from build123d import *

# Parameters (mm, degrees)
F0_R     = 63.5
F1_DEPTH = 254
F2_R     = 31.75
F3_DEPTH = 50.8


# Not quite as in the source:
# - a pattern or mirror of a feature is missing from the dataset's text; its kind, count and spacing are read off the source's solid


with BuildPart() as f1:
    # F0 (on Front) → F1 (new body)
    with BuildSketch(Plane.XZ):
        Circle(F0_R)
    extrude(amount=F1_DEPTH)

    # F2 (on face) → F3 (join)
    with BuildSketch(Plane.XZ.offset(254)):
        Circle(F2_R)
    f3 = extrude(amount=F3_DEPTH)

    # F3_copies: F3 across plane
    add(f3.mirror(Plane.ZX.offset(-127)))


solid = f1.part
Verification items for the finished model (mm, model axes). A direction names the side the tool comes from. Coordinates: 2 decimals unless noted, no trailing zeros. Order: outer loops, then holes, each group sorted by start corner. A loop starts at its lowest first (then second) coordinate and runs counter-clockwise, first axis right, second up. Notation, with made-up numbers: M -17,22 L 3,22 A21 cw 3,52 Z; hole C -22,53 d8. An arc over 180 degrees is marked long. One line per item, written item: value. Start each with the question number.
Item 1: Sectioned sample at D-D on x = -47.5. Record the cut outline in (y, z), then the cut area to 3 significant figures.
Item 2: Thickness scan on probe 1 along Z at (x, y) = (-1, -238); probe 2 along Y at (x, z) = (27, 55.5); probe 3 along X at (y, z) = (-133, 1.5). Record the ranges inside material, lowest first.
Item 3: Sectioned sample at C-C on y = -102.5. Record the cut outline in (x, z), then the cut area to 3 significant figures.
Item 4: Access from +Z, -Z, +X, -X, +Y, -Y to the whole of each face (thin tool, end or side, straight path). Record for faces 1 (the flat face through (0, 50.8, 0)), 2 (the cylindrical face through (-6.883, -279.044, -30.995)), 3 (the flat face through (13.2, 0, 29.1)).
Item 5: Sectioned sample at B-B on x = 0. Record the cut outline in (y, z).
Item 6: Sectioned sample at A-A on z = 0. Record the cut outline in (x, y), then the cut area to 3 significant figures.
Item 7: Depth check by flat-ended pin: P1, Ø3, axis at y = -63.5, z = 22.5, coming from the +X side; P2, Ø5, axis at x = -28.5, z = 47.5, coming from the +Y side; P3, Ø1, axis at x = -44.5, y = -189, coming from the -Z side. Enter the tip coordinate at first touch or a pass-through.
Calculated:
1. outline: M -254,-42.14 L 0,-42.14 L 0,42.14 L -254,42.14 Z
1. area: 21,400 mm^2
2. probe 1: -63.49 to 63.49
2. probe 2: -254 to 0
2. probe 3: -63.48 to 63.48
3. outline: C 0,0 d127
3. area: 12,700 mm^2
4. face 1: +Z, -Z, +X, -X, +Y
4. face 2: -Y
4. face 3: +Y
5. outline: M -304.8,-31.75 L -254,-31.75 L -254,-63.5 L 0,-63.5 L 0,-31.75 L 50.8,-31.75 L 50.8,31.75 L 0,31.75 L 0,63.5 L -254,63.5 L -254,31.75 L -304.8,31.75 Z
6. outline: M -63.5,-254 L -31.75,-254 L -31.75,-304.8 L 31.75,-304.8 L 31.75,-254 L 63.5,-254 L 63.5,0 L 31.75,0 L 31.75,50.8 L -31.75,50.8 L -31.75,0 L -63.5,0 Z
6. area: 38,700 mm^2
7. P1: x = 59.93
7. P2: y = 0
7. P3: z = -45.78
